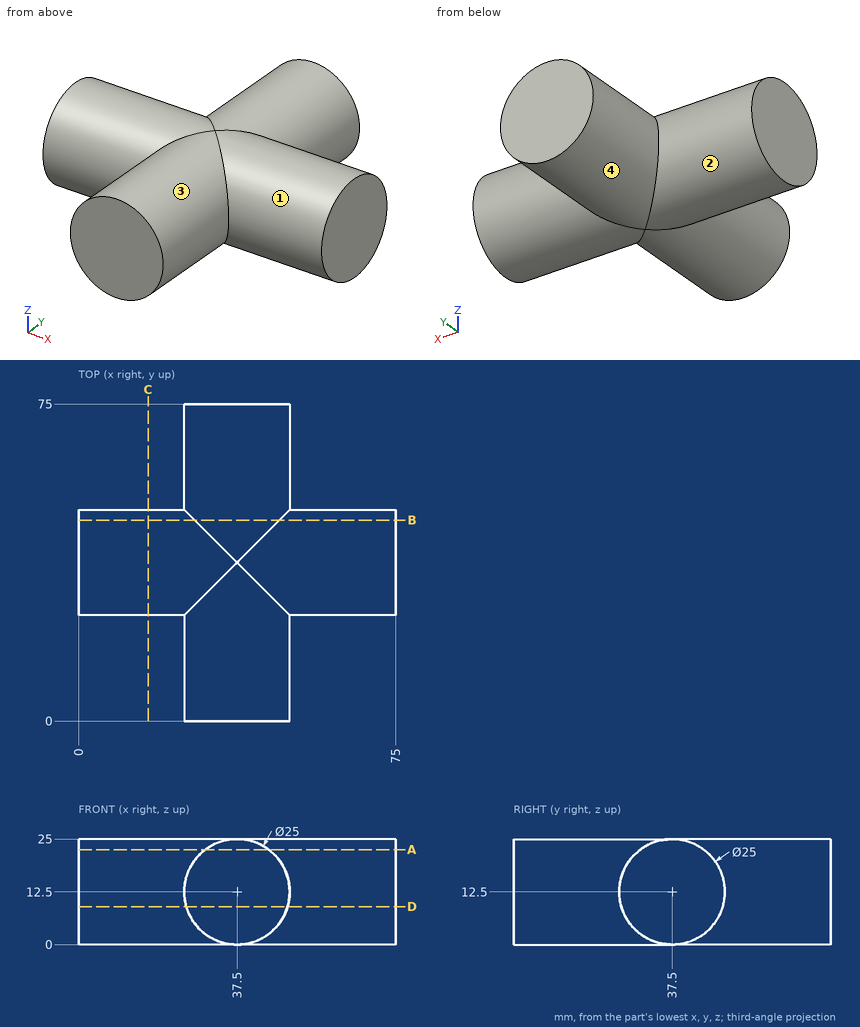
For this review, use the dimensioned drawing (mm, ordinates from the lowest corner) and the shaded views. A direction names the side the tool comes from. Coordinates: 2 decimals unless noted, no trailing zeros. Order: outer loops, then holes, each group sorted by start corner. A loop starts at its lowest first (then second) coordinate and runs counter-clockwise, first axis right, second up. Notation, with made-up numbers: (55, 62) -> (86, 62) arc R10 ccw to (86, 77) -> close; hole circle Ø4 at (17.25, 9.5). An arc over 180 degrees is marked (long way). One line per item, written item: value. Start each with the question number.
Q1. Take a section at D-D, the plane z = 9. State the section outline as (x, y) points.
Q2. Take a section at C-C, the plane x = 16.5. State the section outline as (y, z) points, then the cut area to 3 significant figures.
Q3. Tool access review of the marked faces 1, 2, 3 and 4: name each direction out of +Z, -Z, +X, -X, +Y, -Y from which nothing blocks a thin tool from reaching the whole face with its end or side.
Q4. Take a section at B-B, the plane y = 47.5. State the section outline as (x, z) points.
Q5. Take a section at A-A, the plane z = 22.5. State the section outline as (x, y) points, then the cut area to 4 significant figures.
Q6. Insertion check: pin 1 Ø4 at (x, y) = (53.5, 26) entering from -Z; pin 2 Ø6 at (y, z) = (65, 9.5) entering from -X; pin 3 Ø5 at (x, y) = (40.5, 26.5) entering from -Z. Each pin has a flat end and moves straight along its axis. Give the tip position at first contact, or say it passes through.
Q7. For probe 1 along Y at (x, z) = (7.5, 11.75); probe 2 along X at (y, z) = (25, 14); probe 3 along Y at (x, z) = (68.5, 19), list the stretches that pass through material, from the lowest coordinate up.
Values follow:
1. outline: (0, 25.5) -> (25.5, 25.5) -> (25.5, 0) -> (49.5, 0) -> (49.5, 25.5) -> (75, 25.5) -> (75, 49.5) -> (49.5, 49.5) -> (49.5, 75) -> (25.5, 75) -> (25.5, 49.5) -> (0, 49.5) -> close
2. outline: circle Ø25 at (37.5, 12.5)
2. area: 491 mm2
3. face 1: +X
3. face 2: -X
3. face 3: -Y
3. face 4: +Y
4. outline: (0, 5) -> (27.5, 5) arc R12.5 ccw to (47.5, 5) -> (75, 5) -> (75, 20) -> (47.5, 20) arc R12.5 ccw to (27.5, 20) -> (0, 20) -> close
5. outline: (0, 30) -> (30, 30) -> (30, 0) -> (45, 0) -> (45, 30) -> (75, 30) -> (75, 45) -> (45, 45) -> (45, 75) -> (30, 75) -> (30, 45) -> (0, 45) -> close
5. area: 2,025 mm2
6. pin 1: stops at z = 4.38
6. pin 2: stops at x = 25
6. pin 3: stops at z = 0.01
7. probe 1: y = 25.02 to 49.98
7. probe 2: x = 25.09 to 49.91
7. probe 3: y = 26.82 to 48.18
